The listing builds one solid part. Answer for the finished solid, in the listing's coordinates (mm). Face numbers are marked on the shaded views. A direction names the side the tool comes from. Give positions to 0.01 mm unless a question says otherwise; leave off trailing zeros. Order: outer loops, then holes, each group sorted by start corner. A loop starts at its lowest first (then second) coordinate and runs counter-clockwise, first axis right, second up. Notation, with made-up numbers: M -15,22 L 28,22 A28 ccw 28,47 Z; hole C 12,65.25 d2. An arc over 180 degrees is marked long. Answer as a JSON object with one key per item and string values. Group by question number.
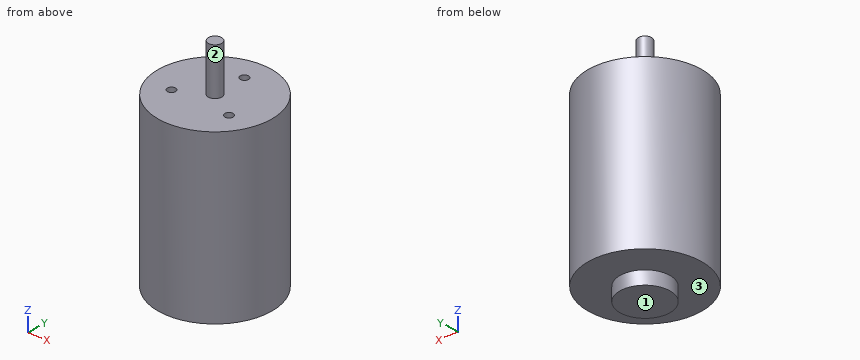
```python
from build123d import *

# Parameters (mm, degrees)
SKETCH1_R                 = 34
BOSS_EXTRUDE1_DEPTH       = 100
SKETCH3_R                 = 4
BOSS_EXTRUDE2_DEPTH       = 28
M6X1_0_TAPPED_HOLE1_D     = 5
M6X1_0_TAPPED_HOLE1_DEPTH = 14.9987
M6X1_0_TAPPED_HOLE1_TIP   = 1.502151548
SKETCH6_R                 = 15
BOSS_EXTRUDE3_DEPTH       = 8


with BuildPart() as part:
    # Sketch1 → Boss-Extrude1 (new body)
    with BuildSketch(Plane.XY):
        Circle(SKETCH1_R)
    extrude(amount=BOSS_EXTRUDE1_DEPTH)

    # Sketch3 → Boss-Extrude2 (add)
    with BuildSketch(Plane.XY.offset(100)):
        Circle(SKETCH3_R)
    extrude(amount=BOSS_EXTRUDE2_DEPTH)

    # M6x1.0 Tapped Hole1
    with Locations(Plane(origin=(0, 20, 100), x_dir=(1, 0, 0), z_dir=(0, 0, 1))):
        with Locations((0, 0), (17.320508076, -30), (-17.320508076, -30)):
            Hole(M6X1_0_TAPPED_HOLE1_D / 2, depth=M6X1_0_TAPPED_HOLE1_DEPTH)
            with Locations((0, 0, -(M6X1_0_TAPPED_HOLE1_DEPTH + M6X1_0_TAPPED_HOLE1_TIP / 2))):  # 118° drill point
                Cone(0, M6X1_0_TAPPED_HOLE1_D / 2, M6X1_0_TAPPED_HOLE1_TIP, mode=Mode.SUBTRACT)

    # Sketch6 → Boss-Extrude3 (add)
    with BuildSketch(Plane(origin=(0, 0, 0), x_dir=(-1, 0, 0), z_dir=(0, 0, -1))):
        with Locations(Location((0, 0, 0), (0, 0, 180))):
            Circle(SKETCH6_R)
    extrude(amount=BOSS_EXTRUDE3_DEPTH)


solid = part.part
```
Item 1: Flat-ended cylindrical pins translate along their axes: P1, Ø8, axis at x = -21.5, z = 68.5, coming from the -Y side; P2, Ø1, axis at x = 3.5, z = 106.5, coming from the +Y side; P3, Ø4, axis at x = 0, y = 20, coming from the -Z side. Find the tip coordinate at first contact, or state that the pin passes through.
Item 2: Section C-C (z = 117.5) is taken. Determine the outline of the cut face in (x, y).
Item 3: Section A-A (y = 0) is taken. Determine the outline of the cut face in (x, z).
Item 4: Section D-D (x = 9) is taken. Determine the outline of the cut face in (y, z).
Item 5: Section B-B (x = -6.5) is taken. Determine the outline of the cut face in (y, z), and give its area (3 significant figures).
Item 6: A tool of negligible diameter and unlimited length cuts with its end or side. For the marked faces 1, 2 and 3, from which of +Z, -Z, +X, -X, +Y, -Y can it reach the whole face along a straight path? Write none if from no direction.
Item 7: Consider probe 1 along Z at (x, y) = (14.5, 24.5); probe 2 along Y at (x, z) = (-0.5, 48.5); probe 3 along X at (y, z) = (20, 95.5). Determine where each line is inside the solid, lowest interval first. Write a range as from..to.
Values found:
{
 "1": {"P1": "stops at y = -29.15", "P2": "stops at y = 2.65", "P3": "stops at z = 0"},
 "2": {"outline": "C 0,0 d8"},
 "3": {"outline": "M -34,0 L -15,0 L -15,-8 L 15,-8 L 15,0 L 34,0 L 34,100 L 4,100 L 4,128 L -4,128 L -4,100 L -34,100 Z"},
 "4": {"outline": "M -32.79,0 L -12,0 L -12,-8 L 12,-8 L 12,0 L 32.79,0 L 32.79,100 L -32.79,100 Z"},
 "5": {"outline": "M -33.37,0 L -13.52,0 L -13.52,-8 L 13.52,-8 L 13.52,0 L 33.37,0 L 33.37,100 L -33.37,100 Z", "area": "6,890 mm^2"},
 "6": {"face 1": "-Z, +X, -X, +Y, -Y", "face 2": "+Z", "face 3": "-Z"},
 "7": {"probe 1": "z = 0..100", "probe 2": "y = -34..34", "probe 3": "x = -27.5..-2.5, 2.5..27.5"}
}
